Answer from the drawing. Dimensions are ordinates in mm from the lowest x, y and z of the part. A direction names the side the tool comes from. Give positions to 0.01 mm unless a question says otherwise; leave off trailing zeros. Write each loop counter-clockwise with the first axis right and the second up, starting at its lowest first coordinate (ties: lowest second). Pieces come first, ordered by that corner, then holes. Notation, with made-up numbers: (21, -14) -> (69, -14) arc R24 ccw to (69, 8) -> close; hole circle Ø4 at (75.5, 77). An arc over 180 degrees is marked (long way). Use a Markdown table: item, result. Add a question column.
Q1. Section C-C, the plane z = 51 is taken. Give the vertices of the cut face in (x, y), plus the area to 3 significant figures.
Q2. Consider line 1 (Y direction, x = 254, z = 28); line 2 (Y direction, x = 45, z = 52.5); line 3 (X direction, y = 57.5, z = 138). Determine where each line is inside the solid, lowest interval first.
Q3. Each of these flat-tipped pins is pushed along its axis until it touches: pin 1 Ø2 at (y, z) = (150, 100.5) entering from +X; pin 2 Ø4 at (x, y) = (95, 42) entering from +Z; pin 3 Ø2 at (y, z) = (97.5, 102.5) entering from -X. Where does it stop, or does it pass through?
Q4. For the marked faces 1, 2 and 3, determine the directions among +Z, -Z, +X, -X, +Y, -Y from which every point of the face is accessible in a straight line to the end or side of a thin tool.
Q5. Section B-B, the plane y = 152.4 is taken. Give the vertices of the cut face in (x, z).
Q6. For a pull along Y with two mould halves and no side action, classify the marked faces 4, 5 and 6 as pulls with the +Y half, pulls with the -Y half, needs draft (parallel to the pull), parting line crosses it, or undercut.
Q7. Section D-D, the plane z = 137.5 is taken. Give the vertices of the cut face in (x, y).
Q8. Section A-A, the plane x = 475.5 is taken. Give the vertices of the cut face in (y, z), plus the area to 3 significant figures.
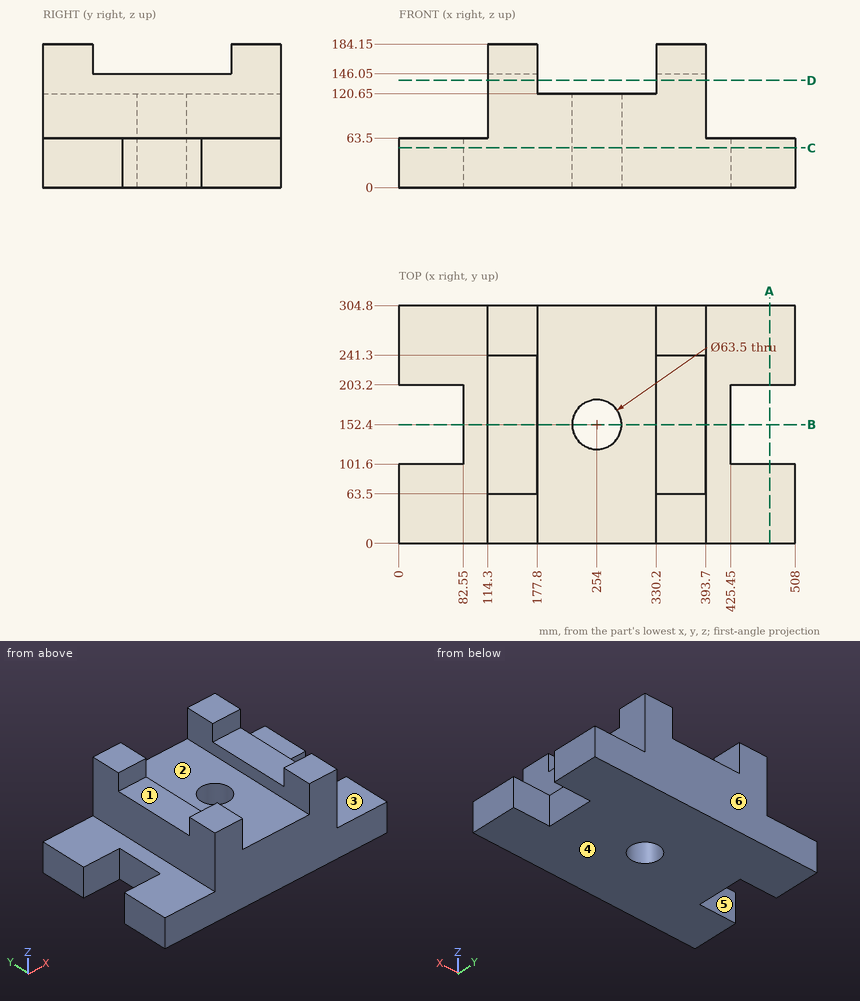
Result set:
| question | item | result |
|---|---|---|
| 1 | outline | (0, 0) -> (508, 0) -> (508, 101.6) -> (425.45, 101.6) -> (425.45, 203.2) -> (508, 203.2) -> (508, 304.8) -> (0, 304.8) -> (0, 203.2) -> (82.55, 203.2) -> (82.55, 101.6) -> (0, 101.6) -> close; hole circle Ø63.5 at (254, 152.4) |
| 1 | area | 135,000 mm2 |
| 2 | line 1 | y = 0 to 120.65, 184.15 to 304.8 |
| 2 | line 2 | y = 0 to 101.6, 203.2 to 304.8 |
| 2 | line 3 | x = 114.3 to 177.8, 330.2 to 393.7 |
| 3 | pin 1 | stops at x = 393.7 |
| 3 | pin 2 | stops at z = 63.5 |
| 3 | pin 3 | stops at x = 114.3 |
| 4 | face 1 | +Z, +X, -X |
| 4 | face 2 | +Z, +Y, -Y |
| 4 | face 3 | +Z, +X, +Y, -Y |
| 5 | outline | (82.55, 0) -> (222.25, 0) -> (222.25, 120.65) -> (177.8, 120.65) -> (177.8, 146.05) -> (114.3, 146.05) -> (114.3, 63.5) -> (82.55, 63.5) -> close; (285.75, 0) -> (425.45, 0) -> (425.45, 63.5) -> (393.7, 63.5) -> (393.7, 146.05) -> (330.2, 146.05) -> (330.2, 120.65) -> (285.75, 120.65) -> close |
| 6 | face 4 | needs draft |
| 6 | face 5 | undercut |
| 6 | face 6 | pulls with the +Y half |
| 7 | outline | (114.3, 0) -> (177.8, 0) -> (177.8, 304.8) -> (114.3, 304.8) -> close; (330.2, 0) -> (393.7, 0) -> (393.7, 304.8) -> (330.2, 304.8) -> close |
| 8 | outline | (0, 0) -> (101.6, 0) -> (101.6, 63.5) -> (0, 63.5) -> close; (203.2, 0) -> (304.8, 0) -> (304.8, 63.5) -> (203.2, 63.5) -> close |
| 8 | area | 12,900 mm2 |
